Can you work these out from the drawing? Everything is in mm from the part's minimum corner. A direction names the side the tool comes from. Round coordinates to 2 decimals unless told otherwise and drop trailing zeros. Write each loop counter-clockwise with the first axis right and the second up, starting at its lowest first coordinate (ties: lowest second). Pieces come first, ordered by that corner, then holes. Notation, with made-up numbers: (78.25, 76) -> (130.25, 76) arc R29 ccw to (130.25, 111) -> close; hole circle Ø3 at (40.25, 65). An arc over 180 degrees is marked (long way). Answer as CSV lines item,"result". Start each with the question number.
Q1. Imagine slicing it at D-D on z = 4.25. Please give me the cut outline in (x, y).
Q2. Will these pins go through, and if not, where does the flat tip stop? pin 1 Ø3 at (x, z) = (9, 21.5) entering from -Y; pin 2 Ø3 at (y, z) = (3.5, 8) entering from +X.
Q3. Imagine slicing it at B-B on x = 7.5. Please give me the cut outline in (y, z), and give its area (3 significant figures).
Q4. If I drill on line 1 (Z direction, x = 5.5, y = 14.25); line 2 (Y direction, x = 7.5, z = 26.15); line 3 (X direction, y = 5, z = 2.05), over which ranges is the centre line in solid material (lowest first)? Write a range as [from, to].
Q5. If we mould it in two halves opening along Z, with no side actions, what happens to the marked faces 1, 2 and 3? For each: pulls with the +Z half, pulls with the -Z half, needs draft (parallel to the pull), parting line crosses it, or undercut.
Q6. Imagine slicing it at C-C on y = 5. Please give me the cut outline in (x, z), and give its area (3 significant figures).
Q7. For the marked faces 4 and 5, which set-ups out of +Z, -Z, +X, -X, +Y, -Y let a thin tool reach every point of the face, with its end or its side?
Q8. Imagine slicing it at A-A on y = 9.25. Please give me the cut outline in (x, z).
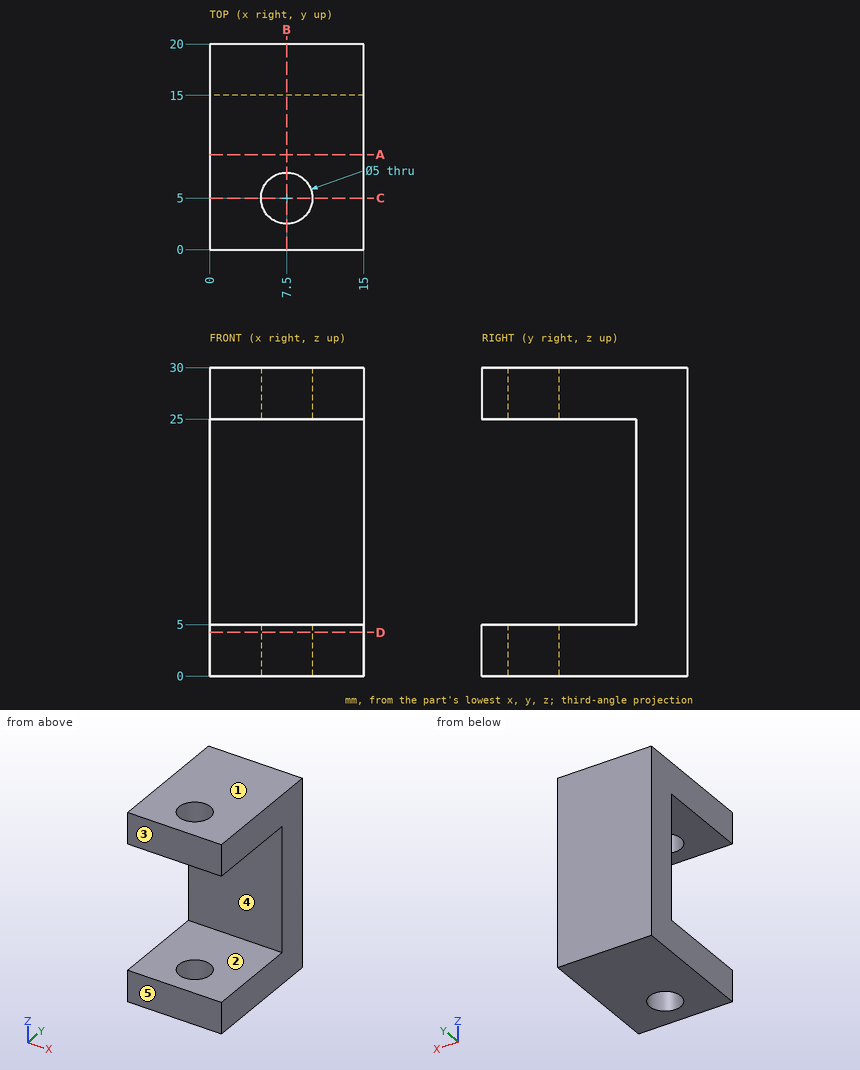
Checks:
1,outline,"(0, 0) -> (15, 0) -> (15, 20) -> (0, 20) -> close; hole circle Ø5 at (7.5, 5)"
2,pin 1,"y = 15"
2,pin 2,"through"
3,outline,"(0, 0) -> (2.5, 0) -> (2.5, 5) -> (0, 5) -> close; (0, 25) -> (2.5, 25) -> (2.5, 30) -> (0, 30) -> close; (7.5, 0) -> (20, 0) -> (20, 30) -> (7.5, 30) -> (7.5, 25) -> (15, 25) -> (15, 5) -> (7.5, 5) -> close"
3,area,"250 mm^2"
4,line 1,"[0, 5], [25, 30]"
4,line 2,"[0, 2.5], [7.5, 20]"
4,line 3,"[0, 5], [10, 15]"
5,face 1,"pulls with the +Z half"
5,face 2,"undercut"
5,face 3,"needs draft"
6,outline,"(0, 0) -> (5, 0) -> (5, 5) -> (0, 5) -> close; (0, 25) -> (5, 25) -> (5, 30) -> (0, 30) -> close; (10, 0) -> (15, 0) -> (15, 5) -> (10, 5) -> close; (10, 25) -> (15, 25) -> (15, 30) -> (10, 30) -> close"
6,area,"100 mm^2"
7,face 4,"+X, -X, -Y"
7,face 5,"+Z, -Z, +X, -X, -Y"
8,outline,"(0, 0) -> (15, 0) -> (15, 5) -> (0, 5) -> close; (0, 25) -> (15, 25) -> (15, 30) -> (0, 30) -> close"
